from build123d import *

# Parameters (mm, degrees)
F1_DEPTH  = 31.75
F2_W      = 2.54
F2_H      = 18.923
F3_DEPTH  = 31.75
F5_DEPTH  = 2.54
F6_W      = 10.16
F6_H      = 5.08
F7_DEPTH  = 10.16
F8_R      = 1.27
F9_R      = 2.54
F10_DEPTH = 5.08


with BuildPart() as f1:
    # F0 (on Front) → F1 (new body, symmetric)
    with BuildSketch(Plane.XZ):
        Polygon((-19.05, -13.97), (19.05, -13.97), (19.05, 13.97), (15.875, 13.97), (15.875, 11.43), (17.145, 11.43), (17.145, 8.128), (15.875, 8.128), (15.875, -10.795), (0, -10.795), (-15.875, -10.795), (-15.875, 8.128), (-17.145, 8.128), (-17.145, 11.43), (-15.875, 11.43), (-15.875, 13.97), (-19.05, 13.97), align=None)
    extrude(amount=F1_DEPTH, both=True)

    # F2 (on face) → F3 (join, through all)
    with BuildSketch(Plane(origin=(15.875, 0, 0), x_dir=(0, -1, 0), z_dir=(-1, 0, 0))):
        with Locations((-30.48, -1.3335)):
            Rectangle(F2_W, F2_H)
        with Locations((30.48, -1.3335)):
            Rectangle(F2_W, F2_H)
    extrude(amount=F3_DEPTH)

    # F4 (on face) → F5 (cut, through all)
    with BuildSketch(Plane.XZ.offset(31.75)):
        with BuildLine():
            ThreePointArc((-1.034546, 8.128), (0, 7.093454), (1.034546, 8.128))
            Line((1.034546, 8.128), (-1.034546, 8.128))
        make_face()
    extrude(amount=-F5_DEPTH, mode=Mode.SUBTRACT)

    # F6 (on face) → F7 (join)
    with BuildSketch(Plane.XY.offset(-10.795)):
        with Locations((0, -21.59)):
            Rectangle(F6_W, F6_H)
    extrude(amount=F7_DEPTH)

    # F8
    f8_edges = [f1.edges().sort_by_distance(p)[0] for p in [
        (19.05, 31.75, 0),
        (19.05, 0, 13.97),
        (19.05, -31.75, 0),
        (19.05, 0, -13.97),
        (0, -31.75, -13.97),
        (-19.05, -31.75, 0),
        (-19.05, 0, 13.97),
        (-19.05, 31.75, 0),
        (-19.05, 0, -13.97),
        (0, 31.75, -13.97),
        (0, -19.05, -0.635),
        (-5.08, -21.59, -0.635),
        (-5.08, -19.05, -5.715),
        (0, -24.13, -0.635),
        (5.08, -21.59, -0.635),
        (5.08, -24.13, -5.715),
        (5.08, -19.05, -5.715),
        (-5.08, -24.13, -5.715),
        (-15.875, 0, 13.97),
        (15.875, 0, 13.97),
        (17.4625, -31.75, 13.97),
        (-17.4625, -31.75, 13.97),
        (-17.4625, 31.75, 13.97),
        (17.4625, 31.75, 13.97),
    ]]
    fillet(f8_edges, radius=F8_R)

    # F9 (on face) → F10 (cut, through all)
    with BuildSketch(Plane(origin=(0, -19.05, 0), x_dir=(-1, 0, 0), z_dir=(0, 1, 0))):
        with Locations((0, -6.35)):
            Circle(F9_R)
    extrude(amount=-F10_DEPTH, mode=Mode.SUBTRACT)


solid = f1.part
Check sheet for the modelled part. Datum: model origin and axes. Units: mm. A direction names the side the tool comes from. Round coordinates to 2 decimals unless told otherwise and drop trailing zeros. Order: outer loops, then holes, each group sorted by start corner. A loop starts at its lowest first (then second) coordinate and runs counter-clockwise, first axis right, second up. Notation, with made-up numbers: M 47,12 L 52,12 A10 ccw 52,31 Z; hole C 8.5,54.5 d3. An arc over 180 degrees is marked long. One line per item, written item: value. Start each with the question number.
1. Release check for a two-part mould opening along Y. For faces 1 (the cylindrical face through (0.05, -23.77, -1.02)), 2 (the flat face through (0, -31.75, -3)), 3 (the cylindrical face through (17.026, 31.528, 13.417)) record: released by +Y, released by -Y, zero draft, split by the parting line, or undercut.
2. Gauge pin test, flat ends, axial feed: P1, Ø0.8, axis at x = -2, y = -21.5, coming from the +Z side (3 decimals); P2, Ø1.5, axis at x = 5, y = -13, coming from the +Z side (3 decimals). Record the tip position at first contact, or that the pin passes through.
3. Scan lines: line 1 along Y through (x, z) = (-1.5, -8.5); line 2 along Y through (x, z) = (-9, -9.25); line 3 along Z through (x, y) = (0, -20.65) (3 decimals). Record each from-to range of solid material in increasing order.
4. Section check A-A on z = -6.35. Enter the section's corners in (x, y) (3 decimals), and give its area (3 significant figures).
5. Section check B-B on x = 0. Enter the section's corners in (y, z) (3 decimals).
6. Section check C-C on y = 20.5. Enter the section's corners in (x, z) (3 decimals).
7. Access from +Z, -Z, +X, -X, +Y, -Y to the whole of each face (thin tool, end or side, straight path). Record for faces 4 (the flat face through (-17.145, 0, 10)), 5 (the cylindrical face through (-0.023, -30.498, 7.094)), 6 (the cylindrical face through (-4.698, -19.412, -6.288)), 7 (the cylindrical face through (16.24, -0.44, 13.59)).
8. Section check D-D on z = 3.25. Enter the section's corners in (x, y) (3 decimals), and give its area (3 significant figures).
Results found:
1. face 1: undercut
1. face 2: released by -Y
1. face 3: released by +Y
2. P1: z = -0.635
2. P2: z = -10.795
3. line 1: -31.75 to -29.21, -24.13 to -19.05, 29.21 to 31.75
3. line 2: -31.75 to -29.21, 29.21 to 31.75
3. line 3: -13.97 to -8.89, -3.81 to -0.635
4. outline: M -19.05,-30.48 A1.27 ccw -17.78,-31.75 L 17.78,-31.75 A1.27 ccw 19.05,-30.48 L 19.05,30.48 A1.27 ccw 17.78,31.75 L -17.78,31.75 A1.27 ccw -19.05,30.48 Z; M -5.08,-22.86 A1.27 ccw -3.81,-24.13 L -2.54,-24.13 L -2.54,-19.05 L -3.81,-19.05 A1.27 ccw -5.08,-20.32 Z; M 2.54,-24.13 L 3.81,-24.13 A1.27 ccw 5.08,-22.86 L 5.08,-20.32 A1.27 ccw 3.81,-19.05 L 2.54,-19.05 Z; hole M -15.875,-29.21 L 15.875,-29.21 L 15.875,29.21 L -15.875,29.21 Z
4. area: 588 mm^2
5. outline: M -31.75,-12.7 A1.27 ccw -30.48,-13.97 L 30.48,-13.97 A1.27 ccw 31.75,-12.7 L 31.75,8.128 L 29.21,8.128 L 29.21,-10.795 L -19.05,-10.795 L -19.05,-8.89 L -24.13,-8.89 L -24.13,-10.795 L -29.21,-10.795 L -29.21,7.093 L -31.75,7.093 Z; M -24.13,-3.81 L -19.05,-3.81 L -19.05,-1.905 A1.27 ccw -20.32,-0.635 L -22.86,-0.635 A1.27 ccw -24.13,-1.905 Z
6. outline: M -19.05,-12.7 A1.27 ccw -17.78,-13.97 L 17.78,-13.97 A1.27 ccw 19.05,-12.7 L 19.05,12.7 A1.27 ccw 17.78,13.97 L 17.145,13.97 A1.27 ccw 15.875,12.7 L 15.875,11.43 L 17.145,11.43 L 17.145,8.128 L 15.875,8.128 L 15.875,-10.795 L -15.875,-10.795 L -15.875,8.128 L -17.145,8.128 L -17.145,11.43 L -15.875,11.43 L -15.875,12.7 A1.27 ccw -17.145,13.97 L -17.78,13.97 A1.27 ccw -19.05,12.7 Z
7. face 4: +Y, -Y
7. face 5: +Z, -Y
7. face 6: +Z
7. face 7: +Z, +Y, -Y
8. outline: M -19.05,-30.48 A1.27 ccw -17.78,-31.75 L 17.78,-31.75 A1.27 ccw 19.05,-30.48 L 19.05,30.48 A1.27 ccw 17.78,31.75 L -17.78,31.75 A1.27 ccw -19.05,30.48 Z; hole M -15.875,-29.21 L 15.875,-29.21 L 15.875,29.21 L -15.875,29.21 Z
8. area: 563 mm^2
